Autodesk Inventor part; units mm, degrees
ref_plane "YZ Plane" through (0, 0, 0) normal (1, 0, 0) x (0, 1, 0)
ref_plane "XZ Plane" through (0, 0, 0) normal (0, 1, 0) x (-1, 0, 0)
ref_plane "XY Plane" through (0, 0, 0) normal (0, 0, 1) x (1, 0, 0)
sketch "Sketch1" plane through (0, 0, 0) normal (0, 0, 1) x (1, 0, 0)
  circle A0 centre (0, 0) radius 8
  line L0 (1, 7.9373) -> (40.375, 2.9765)
  line L1 (1, -7.9373) -> (40.375, -2.9765)
  line L2 (0, 0) -> (40, 0) construction
  circle A1 centre (40, 0) radius 3
  circle A2 centre (-10, -17.3205) radius 5
  line L3 (-6.0939, -20.4417) -> (6.2498, -4.994)
  line L4 (-14.6561, -15.4983) -> (-7.4498, 2.9155)
  line L5 (0, 0) -> (-10, -17.3205) construction
  dimension "d0" = 16
  dimension "d1" = 6
  dimension "d2" = 40
  dimension "d3" = 10
  dimension "d4" = 20
  dimension "d5" = 120
extrude "Extrusion1" add sketch "Sketch1" along normal blind 3
fillet "Fillet1" radius 5 1 edges at (4.2224, -7.5313, 1.5)
sketch "Sketch2" plane through (0, 0, 3) normal (0, 0, 1) x (1, 0, 0)
  point P0 (0, 0)
  point P1 (0, 0)
hole "Hole1" at (0, 0, 3) direction (0, 0, -1) diameter 6.2 end through all
sketch "Sketch3" plane through (0, 0, 3) normal (0, 0, 1) x (1, 0, 0)
  arc A0 (-14.6561, -15.4983) -> (-6.0939, -20.4417) centre (-10, -17.3205) ccw
  point P0 (0, 0)
hole "Hole2" at (-10, -17.3205, 3) direction (0, 0, -1) diameter 3.4 end through all
properties part number "Timing_Lever" material "Nylon 6/6"
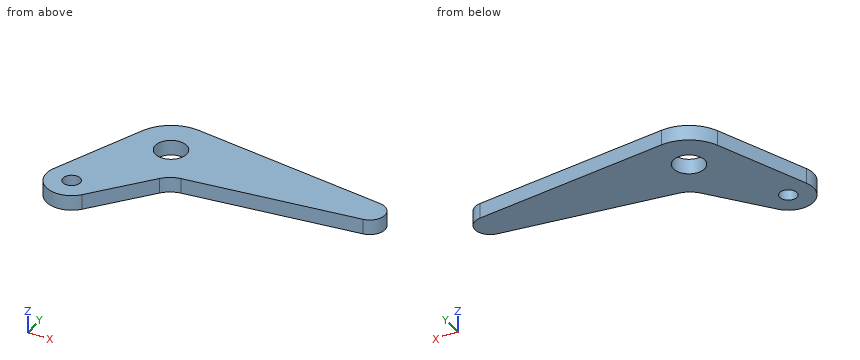
Part model, mm, in its own coordinate system. Round coordinates to 2 decimals unless told otherwise and drop trailing zeros. Write each loop counter-clockwise with the first axis right and the second up, starting at its lowest first coordinate (ties: lowest second). Pieces come first, ordered by that corner, then holes. Notation, with made-up numbers: M 33,56.25 L 47,56.25 A13 cw 47,79.25 Z; hole C 13,66.5 d2. An arc over 180 degrees is marked long. Return JSON: item names as keys, results as strings. Group by question number.
(1) Saw through at C-C on z = 1.4. Write the cut outline in (x, y) (1 decimal).
(2) Saw through at B-B on y = 0. Write the cut outline in (x, z).
(3) Saw through at A-A on x = 2. Write the cut outline in (y, z).
(4) Pin check, flat tips, straight feed: pin 1 Ø1.5 at (x, z) = (14.5, 1) entering from -Y; pin 2 Ø1.5 at (x, z) = (-4.5, 1.5) entering from +Y; pin 3 Ø1.5 at (y, z) = (1.5, 2.5) entering from +X. Stop position of each tip, or through.
(5) Saw through at D-D on y = -6. Write the cut outline in (x, z), then the cut area to 3 significant figures.
(6) Drill centre lines: probe 1 along X at (y, z) = (-17, 2.35); probe 2 along Y at (x, z) = (0, 1.95); probe 3 along X at (y, z) = (0, 0.95). Where is each one in solid material? Low to high.
Returned:
{
 "1": {"outline": "M -14.7,-15.5 A5 ccw -6.1,-20.4 L 3,-9.1 A5 cw 6.2,-7.3 L 40.4,-3 A3 ccw 40.4,3 L 1,7.9 A8 ccw -7.4,2.9 Z; hole C -10,-17.3 d3.4; hole C 0,0 d6.2"},
 "2": {"outline": "M -8.59,0 L -3.1,0 L -3.1,3 L -8.59,3 Z; M 3.1,0 L 43,0 L 43,3 L 3.1,3 Z"},
 "3": {"outline": "M -10.31,0 L -2.37,0 L -2.37,3 L -10.31,3 Z; M 2.37,0 L 7.81,0 L 7.81,3 L 2.37,3 Z"},
 "4": {"pin 1": "y = -6.33", "pin 2": "y = 7.07", "pin 3": "x = 42.9"},
 "5": {"outline": "M -10.94,0 L 16.38,0 L 16.38,3 L -10.94,3 Z", "area": "81.9 mm²"},
 "6": {"probe 1": "-14.99 to -11.67, -8.33 to -3.34", "probe 2": "-12.82 to -3.1, 3.1 to 8", "probe 3": "-8.59 to -3.1, 3.1 to 43"}
}
